```python
from build123d import *

# Parameters (mm, degrees)
F0_W     = 10
F0_H     = 10
F0_R     = 3
F1_DEPTH = 10
F2_DEPTH = 33
F3_SIZE  = 1
F4_R     = 2.5
F5_DEPTH = 25


with BuildPart() as f1:
    # F0 (on Top) → F1 (new body)
    with BuildSketch(Plane.XY):
        Rectangle(F0_W, F0_H)
        Circle(F0_R, mode=Mode.SUBTRACT)
    extrude(amount=F1_DEPTH)

    # F0 (on Top) → F2 (join)
    with BuildSketch(Plane.XY):
        Circle(F0_R)
    extrude(amount=F2_DEPTH)

    # F3
    f3_edges = [f1.edges().sort_by_distance(p)[0] for p in [
        (-3, 0, 33),
    ]]
    chamfer(f3_edges, length=F3_SIZE)

    # F4 (on face) → F5 (cut)
    with BuildSketch(Plane.XZ.offset(5)):
        with Locations((0, 5)):
            Circle(F4_R)
    extrude(amount=-F5_DEPTH, mode=Mode.SUBTRACT)


solid = f1.part
```
For this review, take the finished solid that the model builds, in its own axes (mm). A direction names the side the tool comes from. Round coordinates to 2 decimals unless told otherwise and drop trailing zeros. Write each loop counter-clockwise with the first axis right and the second up, starting at its lowest first coordinate (ties: lowest second). Pieces come first, ordered by that corner, then holes.
1) Mouldability with a two-part tool opening along X and no side actions: class faces 3 (the face through (-0.33, -0.07, 7.48)), 4 (the face through (-2, 5, 3)), 5 (the face through (5, 0, 5)) as +X half, -X half, draft (parallel to the pull), parting line (faces both ways), or undercut.
Answer below:
face 3: undercut
face 4: draft
face 5: +X half
2) Machinability: for faces 1 (the face through (-5, 0, 5)), 2 (the face through (-3, 0, 21)), which of the approach directions +Z, -Z, +X, -X, +Y, -Y give a long, thin tool a straight path to every point of the face, cutting with its end or side? Answer none if there is none.
Answer below:
face 1: +Z, -Z, -X, +Y, -Y
face 2: +Z
3) Take a section at A-A on x = 0. Give the boundary of the cut face in (y, z).
Answer below:
outline: (-5, 0) - (5, 0) - (5, 2.5) - (-5, 2.5) - close; (-5, 7.5) - (5, 7.5) - (5, 10) - (3, 10) - (3, 32) - (2, 33) - (-2, 33) - (-3, 32) - (-3, 10) - (-5, 10) - close
4) Insertion check: pin 1 Ø3 at (x, z) = (0, 5) entering from -Y; pin 2 Ø2 at (x, z) = (-3.5, 18) entering from -Y; pin 3 Ø1.5 at (y, z) = (3, 11.5) entering from -X. Each pin has a flat end and moves straight along its axis. Give the tip position at first contact, or say it passes through.
Answer below:
pin 1: passes through
pin 2: stops at y = -1.66
pin 3: stops at x = -1.98
5) Take a section at C-C on z = 5. Give the boundary of the cut face in (x, y), then the cut area to 3 significant figures.
Answer below:
outline: (-5, -5) - (-2.5, -5) - (-2.5, 5) - (-5, 5) - close; (2.5, -5) - (5, -5) - (5, 5) - (2.5, 5) - close
area: 50.0 mm2
6) For line 1 along Z through (x, y) = (0, 1); line 2 along Z through (x, y) = (1, 0.25); line 3 along Z through (x, y) = (4, -3.5), list the stretches that pass through material, from the lowest coordinate up.
Answer below:
line 1: z = 0 to 2.5, 7.5 to 33
line 2: z = 0 to 2.71, 7.29 to 33
line 3: z = 0 to 10
7) Take a section at D-D on x = -4. Give the boundary of the cut face in (y, z).
Answer below:
outline: (-5, 0) - (5, 0) - (5, 10) - (-5, 10) - close
8) Take a section at B-B on y = 0. Give the boundary of the cut face in (x, z).
Answer below:
outline: (-5, 0) - (5, 0) - (5, 10) - (3, 10) - (3, 32) - (2, 33) - (-2, 33) - (-3, 32) - (-3, 10) - (-5, 10) - close; hole circle Ø5 at (0, 5)
